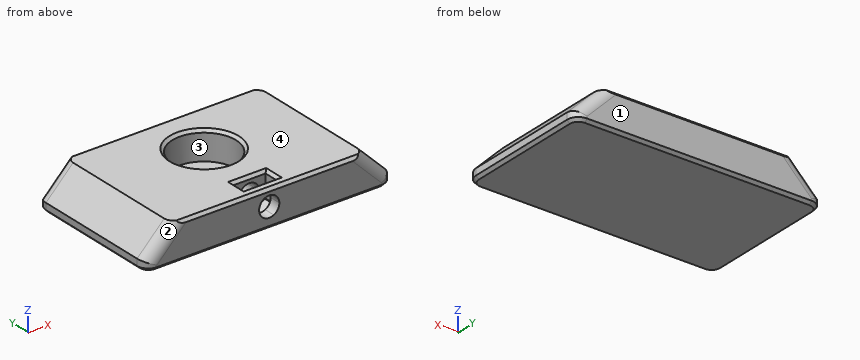
```python
from build123d import *

# Parameters (mm, degrees)
SKIZZE1_W                            = 44
SKIZZE1_H                            = 25
AUFSATZ_LINEAR_AUSTRAGEN1_DEPTH      = 6.5
SKIZZE2_R                            = 5.675
SCHNITT_LINEAR_AUSTRAGEN1_DEPTH      = 5.1
VERRUNDUNG1_R                        = 2
SKIZZE8_W                            = 5.8
SKIZZE8_H                            = 2.6
SCHNITT_LINEAR_AUSTRAGEN5_DEPTH      = 4.5
SCHNITT_LINEAR_AUSTRAGEN6_DEPTH      = 2.6
SCHNITT_LINEAR_AUSTRAGEN7_DEPTH      = 31.698697041
SCHNITT_LINEAR_AUSTRAGEN7_DEPTH_BACK = 4.1
SCHNITT_LINEAR_AUSTRAGEN8_DEPTH      = 34.930075155
FASE1_SIZE                           = 0.5
VERRUNDUNG2_R                        = 2


with BuildPart() as part:
    # Skizze1 → Aufsatz-Linear austragen1 (new body)
    with BuildSketch(Plane.XY):
        with Locations((0, -2.5)):
            Rectangle(SKIZZE1_W, SKIZZE1_H)
    extrude(amount=AUFSATZ_LINEAR_AUSTRAGEN1_DEPTH)

    # Skizze2 → Schnitt-Linear austragen1 (cut)
    with BuildSketch(Plane.XY.offset(6.5)):
        Circle(SKIZZE2_R)
    extrude(amount=-SCHNITT_LINEAR_AUSTRAGEN1_DEPTH, mode=Mode.SUBTRACT)

    # Verrundung1
    verrundung1_edges = [part.edges().sort_by_distance(p)[0] for p in [
        (-22, 10, 3.25),
        (22, 10, 3.25),
        (22, -15, 3.25),
        (-22, -15, 3.25),
    ]]
    fillet(verrundung1_edges, radius=VERRUNDUNG1_R)

    # Skizze8 → Schnitt-Linear austragen5 (cut)
    with BuildSketch(Plane.XY.offset(6.5)):
        with Locations((0, -11.7)):
            Rectangle(SKIZZE8_W, SKIZZE8_H)
    extrude(amount=-SCHNITT_LINEAR_AUSTRAGEN5_DEPTH, mode=Mode.SUBTRACT)

    # Skizze9 → Schnitt-Linear austragen6 (cut)
    with BuildSketch(Plane.XZ.offset(10.4)):
        with BuildLine():
            Line((-0.820441954, 2), (-2.775, 2))
            Line((-2.775, 2), (0, 0.397853003))
            Line((0, 0.397853003), (2.775, 2))
            Line((2.775, 2), (0.820441954, 2))
            ThreePointArc((0.820441954, 2), (0, 1.802146997), (-0.820441954, 2))
        make_face()
        with BuildLine():
            ThreePointArc((1.8, 3.602146997), (-0.938936761, 5.137854573), (-0.820441954, 2))
            Line((-0.820441954, 2), (0.820441954, 2))
            ThreePointArc((0.820441954, 2), (1.535707576, 2.663210236), (1.8, 3.602146997))
        make_face()
        with BuildLine():
            Line((0.820441954, 2), (-0.820441954, 2))
            ThreePointArc((-0.820441954, 2), (0, 1.802146997), (0.820441954, 2))
        make_face()
    extrude(amount=SCHNITT_LINEAR_AUSTRAGEN6_DEPTH, mode=Mode.SUBTRACT)

    # Skizze9<3> → Schnitt-Linear austragen7 (cut, two sides: drawn at the far end of the back side and taken through both)
    with BuildSketch(Plane.XZ.offset(10.4).offset(-SCHNITT_LINEAR_AUSTRAGEN7_DEPTH_BACK)):
        with BuildLine():
            ThreePointArc((1.8, 3.602146997), (-0.938936761, 5.137854573), (-0.820441954, 2))
            Line((-0.820441954, 2), (0.820441954, 2))
            ThreePointArc((0.820441954, 2), (1.535707576, 2.663210236), (1.8, 3.602146997))
        make_face()
        with BuildLine():
            Line((0.820441954, 2), (-0.820441954, 2))
            ThreePointArc((-0.820441954, 2), (0, 1.802146997), (0.820441954, 2))
        make_face()
    extrude(amount=SCHNITT_LINEAR_AUSTRAGEN7_DEPTH + SCHNITT_LINEAR_AUSTRAGEN7_DEPTH_BACK, mode=Mode.SUBTRACT)

    # Skizze10 → Schnitt-Linear austragen8 (cut, through all)
    with BuildSketch(Plane.XZ.offset(15)):
        Polygon((-22, 1.667157288), (-17.167157288, 6.5), (-22, 6.5), align=None)
        Polygon((22, 1.667157288), (22, 6.5), (17.167157288, 6.5), align=None)
    extrude(amount=-SCHNITT_LINEAR_AUSTRAGEN8_DEPTH, mode=Mode.SUBTRACT)

    # Fase1
    fase1_edges = [part.edges().sort_by_distance(p)[0] for p in [
        (-5.675, 0, 6.5),
        (0, 10, 0),
        (-22, -2.5, 0),
        (22, -2.5, 0),
        (0, -15, 0),
        (-21.414213562, -14.414213562, 0),
        (-21.414213562, 9.414213562, 0),
        (21.414213562, -14.414213562, 0),
        (21.414213562, 9.414213562, 0),
        (2.9, -11.7, 6.5),
        (0, -10.4, 6.5),
        (-2.9, -11.7, 6.5),
        (0, -13, 6.5),
        (0, 10, 6.5),
        (0, -15, 6.5),
    ]]
    chamfer(fase1_edges, length=FASE1_SIZE)

    # Verrundung2
    # the kernel refuses this fillet: 2 mm, written as the material it takes off along each edge
    with BuildSketch(Plane(origin=(-23.535533906, 10, 0.131623382), x_dir=(0.7071067811865477, 0, -0.7071067811865477), z_dir=(0.7071067811865476, 0, 0.7071067811865476)), Plane(origin=(14.131623382, 10, 9.535533906), x_dir=(-0.7071067811865476, 0, -0.7071067811865476), z_dir=(0.7071067811865476, 0, -0.7071067811865475)), Plane(origin=(14.131623382, -15, 9.535533906), x_dir=(0, 1, 0), z_dir=(0.7071067811865476, 0, -0.7071067811865475)), Plane(origin=(-23.535533906, -15, 0.131623382), x_dir=(0, 1, 0), z_dir=(0.7071067811865476, 0, 0.7071067811865476))) as verrundung2_piece_1:
        with BuildLine():
            CenterArc((VERRUNDUNG2_R, -VERRUNDUNG2_R), VERRUNDUNG2_R, 90, 90)
            Line((0, -VERRUNDUNG2_R), (0, 0))
            Line((0, 0), (VERRUNDUNG2_R, 0))
        make_face()
    extrude(amount=13.299137803, mode=Mode.SUBTRACT)


solid = part.part
```
Design review of the part built by this model. Coordinates are the model's own, in mm. Face numbers are marked on the shaded views. Coordinates: 2 decimals unless noted, no trailing zeros. Write each loop counter-clockwise with the first axis right and the second up, starting at its lowest first coordinate (ties: lowest second). Pieces come first, ordered by that corner, then holes.
1) Mouldability with a two-part tool opening along Y and no side actions: class the marked faces 1, 2, 3 and 4 as +Y half, -Y half, draft (parallel to the pull), parting line (faces both ways), or undercut.
2) Insertion check: pin 1 (2 mm diameter, centred on y = -12, z = 4, fed in from -X); pin 2 (3.5 mm diameter, centred on x = 1, y = 1.5, fed in from +Z); pin 3 (0.8 mm diameter, centred on y = -12, z = 4.5, fed in from +X). Each pin has a flat end and moves straight along its axis. Give the tip position at first contact, or say it passes through.
3) To check wall thickness, follow L1, parallel to Y at x = 0, z = 2.25 (3 decimals); L2, parallel to Y at x = 0, z = 5.5 (3 decimals); L3, parallel to X at y = -10.75, z = 6. State the ranges of each line that lie inside material, in increasing order.
4) Add section A-A (y = 0). Write out the cut boundary in (x, z) (3 decimals).
Check result:
1. face 1: +Y half
1. face 2: -Y half
1. face 3: undercut
1. face 4: draft
2. pin 1: stops at x = -20.67
2. pin 2: stops at z = 1.4
2. pin 3: stops at x = 19.57
3. L1: y = -6.3 to -5.675, 5.675 to 10
3. L2: y = -15 to -13, -10.4 to -5.675, 5.675 to 10
3. L3: x = -17.67 to -2.9, 2.9 to 17.67
4. outline: (-22, 0.5) - (-21.5, 0) - (21.5, 0) - (22, 0.5) - (22, 1.667) - (17.167, 6.5) - (6.175, 6.5) - (5.675, 6) - (5.675, 1.4) - (-5.675, 1.4) - (-5.675, 6) - (-6.175, 6.5) - (-17.167, 6.5) - (-22, 1.667) - close
